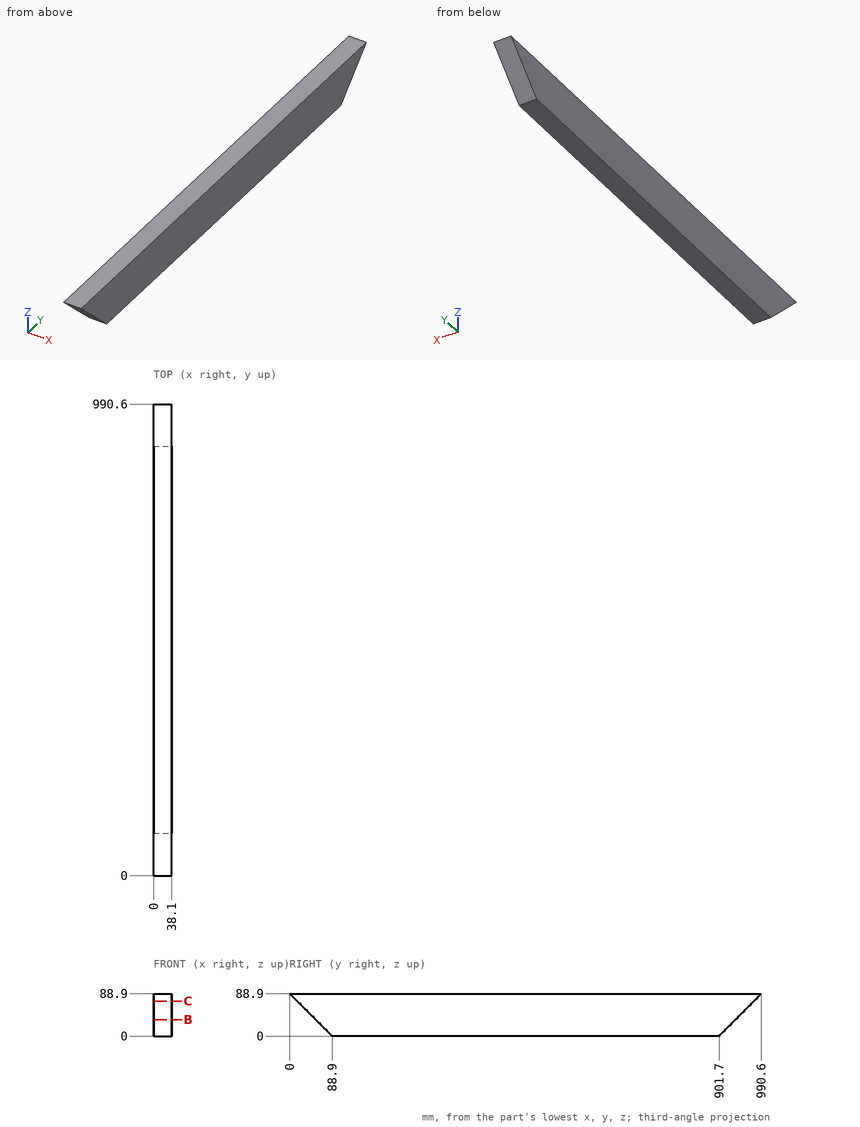
Drawing for the job (mm, zero at the part's lowest x, y, z). Give positions to 0.01 mm unless a question says otherwise; leave off trailing zeros. Order: outer loops, then holes, each group sorted by start corner. A loop starts at its lowest first (then second) coordinate and runs counter-clockwise, first axis right, second up. Notation, with made-up numbers: M 2,29 L 48,29 A21 ccw 48,59 Z; hole C 74.25,39 d5. An arc over 180 degrees is marked long. Write item = value, one per line. Start each with the question number.
(1) Slice it at C-C on z = 73. Write the cut outline in (x, y).
(2) Pin check, flat tip, straight feed: pin 1 Ø6 at (y, z) = (339.5, 43.5) entering from -X. Stop position of the tip, or through.
(3) Slice it at B-B on z = 34.5. Write the cut outline in (x, y), plus the area to 3 significant figures.
(4) Probe L1, parallel to Y at x = 22, z = 62; L2, parallel to Y at x = 8, z = 85. List the from-to ranges inside material, lowest first. Write a range as [from, to].
Responses:
q1.outline = M 0,15.9 L 38.1,15.9 L 38.1,974.7 L 0,974.7 Z
q2.pin_1 = 0
q3.outline = M 0,54.4 L 38.1,54.4 L 38.1,936.2 L 0,936.2 Z
q3.area = 33,600 mm2
q4.L1 = [26.9, 963.7]
q4.L2 = [3.9, 986.7]
